Drawing for the job (mm, zero at the part's lowest x, y, z). A direction names the side the tool comes from. Give positions to 0.01 mm unless a question says otherwise; leave off trailing zeros. Loops run counter-clockwise (first coordinate to the right, second up) from the corner with the lowest first, then second, coordinate; pieces in that order, holes last.
1) Band-saw the part on B-B on z = 55.5. List the corners of the cut face in (x, y).
2) Band-saw the part on C-C on x = 55.5. List the corners of the cut face in (y, z), then the cut area to 3 significant figures.
3) Band-saw the part on D-D on x = 6. List the corners of the cut face in (y, z), then the cut area to 3 significant figures.
4) Two-plate mould, pull along X, no slides. Class the marked faces 1, 2, 3 and 4: +X half, -X half, draft (parallel to the pull), parting line (faces both ways), or undercut.
5) Flat gauge pins, fed straight in: P1, Ø10.5, axis at x = 105, z = 55.5, coming from the +Y side; P2, Ø3, axis at x = 23, y = 11.5, coming from the +Z side; P3, Ø8, axis at x = 16, y = 5.5, coming from the +Z side. Where does each tip first touch, or does it go through?
6) Band-saw the part on A-A on y = 4.75. List the corners of the cut face in (x, z).
7) Wall check: line 1 (X direction, y = 1.5, z = 55.5); line 2 (Z direction, x = 39, y = 14); line 3 (X direction, y = 12, z = 23). Give the ranges that are in metal, low to high.
8) 3-axis set-ups, long thin cutter, end or side, ignore diameter. For the marked faces 5, 6 and 7: which of +Z, -Z, +X, -X, +Y, -Y reach the whole face in a straight line?
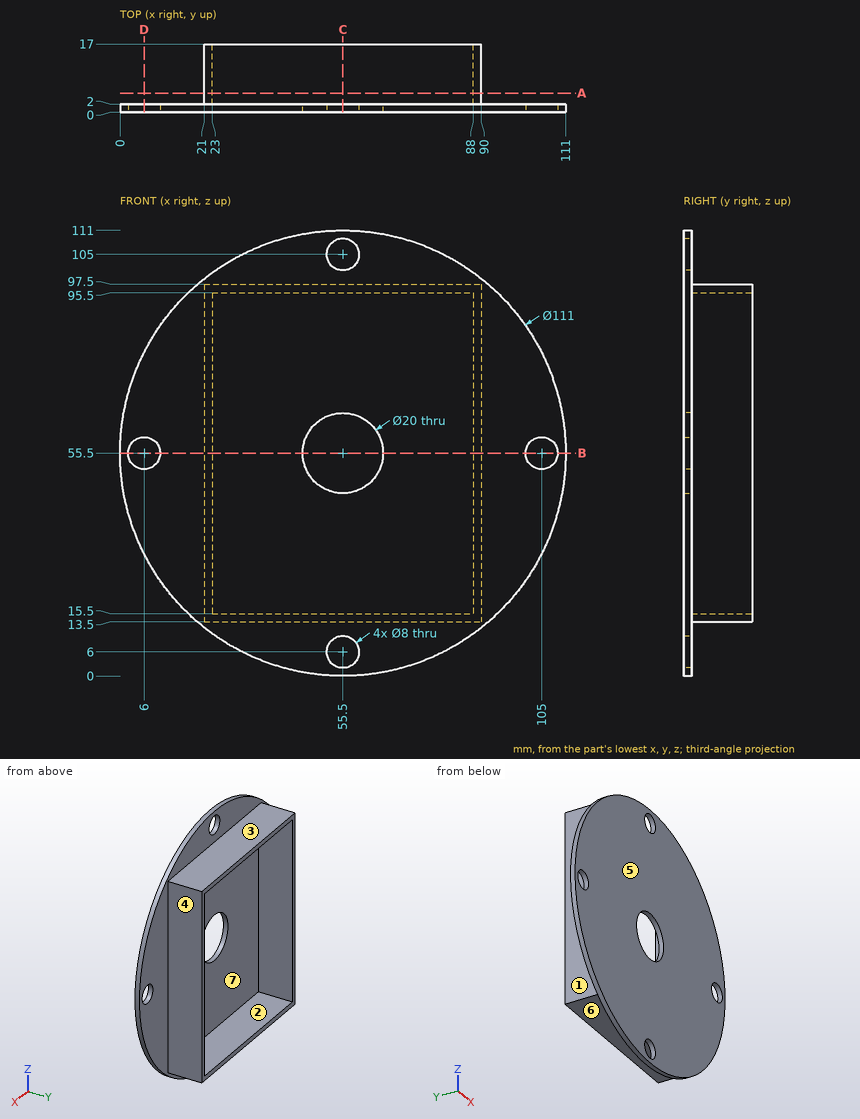
Findings below:
1. outline: (0, 0) - (2, 0) - (2, 2) - (0, 2) - close; (10, 0) - (45.5, 0) - (45.5, 2) - (23, 2) - (23, 17) - (21, 17) - (21, 2) - (10, 2) - close; (65.5, 0) - (101, 0) - (101, 2) - (90, 2) - (90, 17) - (88, 17) - (88, 2) - (65.5, 2) - close; (109, 0) - (111, 0) - (111, 2) - (109, 2) - close
2. outline: (0, 0) - (2, 0) - (2, 2) - (0, 2) - close; (0, 10) - (2, 10) - (2, 13.5) - (17, 13.5) - (17, 15.5) - (2, 15.5) - (2, 45.5) - (0, 45.5) - close; (0, 65.5) - (2, 65.5) - (2, 95.5) - (17, 95.5) - (17, 97.5) - (2, 97.5) - (2, 101) - (0, 101) - close; (0, 109) - (2, 109) - (2, 111) - (0, 111) - close
2. area: 210 mm2
3. outline: (0, 30.4) - (2, 30.4) - (2, 51.5) - (0, 51.5) - close; (0, 59.5) - (2, 59.5) - (2, 80.6) - (0, 80.6) - close
3. area: 84.4 mm2
4. face 1: -X half
4. face 2: undercut
4. face 3: draft
4. face 4: +X half
5. P1: stops at y = 2
5. P2: stops at z = 97.5
5. P3: stops at z = 96.36
6. outline: (21, 13.5) - (90, 13.5) - (90, 97.5) - (21, 97.5) - close; hole (23, 15.5) - (88, 15.5) - (88, 95.5) - (23, 95.5) - close
7. line 1: x = 0 to 2, 10 to 45.5, 65.5 to 101, 109 to 111
7. line 2: z = 13.5 to 15.5, 95.5 to 97.5
7. line 3: x = 21 to 23, 88 to 90
8. face 5: +Z, -Z, +X, -X, -Y
8. face 6: -Z, +X, -X, +Y
8. face 7: +Y
